from build123d import *

# Parameters (mm, degrees)
SKETCH7_W                      = 7
SKETCH7_H                      = 16
BOSS_EXTRUDE6_DEPTH            = 2
SKETCH8_W                      = 2
SKETCH8_H                      = 7.5
BOSS_EXTRUDE7_DEPTH            = 8.5
F_2_2_2_2_DIAMETER_HOLE1_D     = 2.2
F_2_2_2_2_DIAMETER_HOLE1_DEPTH = 2
CUT_EXTRUDE3_DEPTH             = 5.5
CUT_EXTRUDE5_DEPTH             = 10
SKETCH18_W                     = 0.05
SKETCH18_H                     = 16
CUT_EXTRUDE6_DEPTH             = 3


with BuildPart() as part:
    # Sketch7 → Boss-Extrude6 (new body)
    with BuildSketch(Plane.XY):
        with Locations((-14.956904704, 13.340209502)):
            Rectangle(SKETCH7_W, SKETCH7_H)
    extrude(amount=BOSS_EXTRUDE6_DEPTH)

    # Sketch8 → Boss-Extrude7 (add)
    with BuildSketch(Plane(origin=(0, 0, 0), x_dir=(-1, 0, 0), z_dir=(0, 0, -1))):
        with Locations((14.956904704, 17.590209502)):
            Rectangle(SKETCH8_W, SKETCH8_H)
    extrude(amount=BOSS_EXTRUDE7_DEPTH)

    # Ø2.2 (2.2) Diameter Hole1
    with Locations(Plane(origin=(0, 0, 0), x_dir=(-1, 0, 0), z_dir=(0, 0, -1))):
        with Locations((14.956904704, 11.340209502)):
            Hole(F_2_2_2_2_DIAMETER_HOLE1_D / 2, depth=F_2_2_2_2_DIAMETER_HOLE1_DEPTH)

    # Sketch15 → Cut-Extrude3 (cut, through all)
    with BuildSketch(Plane(origin=(-13.956904704, 0, 0), x_dir=(0, 0, -1), z_dir=(1, 0, 0))):
        with BuildLine():
            Line((2.9, 16.640209502), (2.9, 18.640209502))
            ThreePointArc((2.9, 18.640209502), (4.5, 20.240209502), (6.1, 18.640209502))
            Line((6.1, 18.640209502), (6.1, 16.640209502))
            ThreePointArc((6.1, 16.640209502), (4.5, 15.040209502), (2.9, 16.640209502))
        make_face()
    extrude(amount=-CUT_EXTRUDE3_DEPTH, mode=Mode.SUBTRACT)

    # Sketch17 → Cut-Extrude5 (cut)
    with BuildSketch(Plane(origin=(0, 0, 0), x_dir=(-1, 0, 0), z_dir=(0, 0, -1))):
        with BuildLine():
            Line((13.856904704, 7.040209502), (13.856904704, 11.340209502))
            Line((13.856904704, 11.340209502), (16.056904704, 11.340209502))
            Line((16.056904704, 11.340209502), (16.056904704, 7.040209502))
            ThreePointArc((16.056904704, 7.040209502), (14.956904704, 5.940209502), (13.856904704, 7.040209502))
        make_face()
    extrude(amount=-CUT_EXTRUDE5_DEPTH, mode=Mode.SUBTRACT)

    # Sketch18 → Cut-Extrude6 (cut, through all)
    with BuildSketch(Plane(origin=(0, 0, 0), x_dir=(-1, 0, 0), z_dir=(0, 0, -1))):
        with Locations((11.481904704, 13.340209502)):
            Rectangle(SKETCH18_W, SKETCH18_H)
        with Locations((18.431904704, 13.340209502)):
            Rectangle(SKETCH18_W, SKETCH18_H)
    extrude(amount=-CUT_EXTRUDE6_DEPTH, mode=Mode.SUBTRACT)


solid = part.part
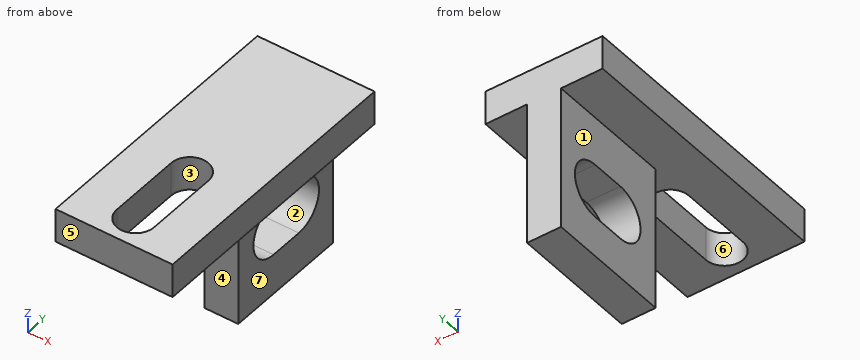
Could you check a few things on this model? Use its own coordinates, in mm. Face numbers are marked on the shaded views. A direction names the side the tool comes from. Coordinates: 2 decimals unless noted, no trailing zeros. Loops run counter-clockwise (first coordinate to the right, second up) from the corner with the lowest first, then second, coordinate; pieces in that order, holes last.
1. For the marked faces 1, 2, 3 and 4, which set-ups out of +Z, -Z, +X, -X, +Y, -Y let a thin tool reach every point of the face, with its end or its side?
2. I need wall thicknesses on L1, parallel to X at y = 8.75, z = 0.75; L2, parallel to Y at x = -14.5, z = -4.5; L3, parallel to Z at x = -13.25, y = 18. Which ranges of each line are inside material? Lowest first, please.
3. Imagine slicing it at C-C (x = -14.75). Please give me the cut outline in (y, z), and give its area (3 significant figures).
4. We'd pull the mould along X, two halves only. Please class the marked faces 5, 6 and 7: released by +X, released by -X, zero draft, split by the parting line, or undercut.
5. Imagine slicing it at B-B (y = 7.25). Please give me the cut outline in (x, z), and give its area (3 significant figures).
6. For P1, Ø1, axis at x = -15.5, z = -3, coming from the -Y side; P2, Ø6, axis at y = 19, z = -7, coming from the -X side; P3, Ø6, axis at y = 19.5, z = -4, coming from the +X side, each with a flat end and sliding along its axis, tell me the tip position at first contact or that it passes through.
7. Imagine slicing it at A-A (z = -4.5). Please give me the cut outline in (x, y).
8. Imagine slicing it at D-D (x = -17.5). Please give me the cut outline in (y, z).
Computed values:
1. face 1: -Z, -X, +Y, -Y
1. face 2: +X, -X
1. face 3: +Z, -Z
1. face 4: -Z, +X, -X, -Y
2. L1: x = -18.41 to -16.06, -13.86 to -11.51
2. L2: y = 13.84 to 15.04, 20.24 to 21.34
2. L3: z = 0 to 2
3. outline: (5.34, 0) - (5.96, 0) - (5.96, 2) - (5.34, 2) - close; (12.42, 0) - (13.84, 0) - (13.84, -8.5) - (21.34, -8.5) - (21.34, 2) - (12.42, 2) - close; hole (16.64, -6.1) - (18.64, -6.1) arc R1.6 ccw to (18.64, -2.9) - (16.64, -2.9) arc R1.6 ccw to start
3. area: 68.4 mm2
4. face 5: zero draft
4. face 6: undercut
4. face 7: released by +X
5. outline: (-18.41, 0) - (-16.06, 0) - (-16.06, 2) - (-18.41, 2) - close; (-13.86, 0) - (-11.51, 0) - (-11.51, 2) - (-13.86, 2) - close
5. area: 9.40 mm2
6. P1: stops at y = 13.84
6. P2: stops at x = -15.96
6. P3: stops at x = -13.96
7. outline: (-15.96, 13.84) - (-13.96, 13.84) - (-13.96, 15.04) - (-15.96, 15.04) - close; (-15.96, 20.24) - (-13.96, 20.24) - (-13.96, 21.34) - (-15.96, 21.34) - close
8. outline: (5.34, 0) - (21.34, 0) - (21.34, 2) - (5.34, 2) - close
